from build123d import *

# Parameters (mm, degrees)
F0_W     = 140
F0_H     = 160
F1_DEPTH = 3.5
F2_W     = 31.75
F2_H     = 31.75
F2_W_2   = 25.4
F2_H_2   = 25.4
F3_DEPTH = 160
F4_W     = 25.4
F4_H     = 25.4
F4_W_2   = 19.4
F4_H_2   = 19.4
F5_DEPTH = 15
F6_R     = 3
F7_DEPTH = 4
F8_R     = 1
F9_DEPTH = 5


with BuildPart() as f1:
    # F0 (on Top) → F1 (new body)
    with BuildSketch(Plane.XY):
        with Locations((-1.276044, 37.026612)):
            Rectangle(F0_W, F0_H)
    extrude(amount=F1_DEPTH)

    # F2 (on face) → F3 (join)
    with BuildSketch(Plane.XZ.offset(42.973388)):
        with Locations((-55.401044, -15.875)):
            Rectangle(F2_W, F2_H)
        with Locations((-55.401044, -15.875)):
            Rectangle(F2_W_2, F2_H_2, mode=Mode.SUBTRACT)
        with Locations((52.848956, -15.875)):
            Rectangle(F2_W, F2_H)
        with Locations((52.848956, -15.875)):
            Rectangle(F2_W_2, F2_H_2, mode=Mode.SUBTRACT)
    extrude(amount=-F3_DEPTH)

    # F4 (on face) → F5 (join, symmetric)
    with BuildSketch(Plane.XZ.offset(42.973388)):
        with Locations((-55.401044, -15.875)):
            Rectangle(F4_W, F4_H)
        with Locations((-55.401044, -15.875)):
            Rectangle(F4_W_2, F4_H_2, mode=Mode.SUBTRACT)
        with Locations((52.848956, -15.875)):
            Rectangle(F4_W, F4_H)
        with Locations((52.848956, -15.875)):
            Rectangle(F4_W_2, F4_H_2, mode=Mode.SUBTRACT)
    extrude(amount=F5_DEPTH, both=True)

    # F6 (on face) → F7 (cut)
    with BuildSketch(Plane.YZ.offset(-39.526044)):
        with Locations((37.026612, -21.75)):
            Circle(F6_R)
    extrude(amount=-F7_DEPTH, mode=Mode.SUBTRACT)

    # F8 (on face) → F9 (cut)
    with BuildSketch(Plane.XY.offset(3.5)):
        with Locations((-66.276044, 112.026612)):
            Circle(F8_R)
        with Locations((63.723956, 112.026612)):
            Circle(F8_R)
        with Locations((63.723956, -37.973388)):
            Circle(F8_R)
        with Locations((-66.276044, -37.973388)):
            Circle(F8_R)
    extrude(amount=-F9_DEPTH, mode=Mode.SUBTRACT)


solid = f1.part
Design review of the part built by this model. Coordinates are the model's own, in mm. A direction names the side the tool comes from. Give positions to 0.01 mm unless a question says otherwise; leave off trailing zeros. Loops run counter-clockwise (first coordinate to the right, second up) from the corner with the lowest first, then second, coordinate; pieces in that order, holes last. Notation, with made-up numbers: (22, -24.75) - (70, -24.75) arc R21 cw to (70, -5.75) - close; hole circle Ø1 at (44.25, 51). An arc over 180 degrees is marked (long way). Write item = value, one per line.
1) Take a section at D-D on x = 0. State the section outline as (y, z) points, and give its area (3 significant figures).
Result sheet:
outline = (-42.97, 0) - (117.03, 0) - (117.03, 3.5) - (-42.97, 3.5) - close
area = 560 mm2
2) Clearance check with flat-ended pins moving along their axes: pin 1 Ø9.5 at (x, y) = (-54, -45.5) entering from +Z; pin 2 Ø7.5 at (x, y) = (46.5, -49) entering from -Z (3 decimals); pin 3 Ø2 at (x, z) = (35, -13) entering from +Y; pin 4 Ø0.6 at (x, y) = (63.5, 111.5) entering from +Z. State where each tip first meets the part, or that it passes through.
Result sheet:
pin_1 = 3.5
pin_2 = -28.575
pin_3 = through
pin_4 = -1.5
3) Take a section at A-A on z = -12.5. Count the separate pieces of the cut face and the enclosed holes in it, and give its area (3 significant figures).
Result sheet:
separate_pieces = 4
enclosed_holes = 0
area = 2,390 mm2
4) To check wall thickness, follow line 1 (X direction, y = 36, z = -19); line 2 (X direction, y = -50, z = -13); line 3 (X direction, y = 3.5, z = -10). State the ranges of each line that lie inside material, in increasing order.
Result sheet:
line_1 = -71.28 to -68.1, 36.97 to 40.15, 65.55 to 68.72
line_2 = -68.1 to -65.1, -45.7 to -42.7, 40.15 to 43.15, 62.55 to 65.55
line_3 = -71.28 to -68.1, -42.7 to -39.53, 36.97 to 40.15, 65.55 to 68.72
5) Draft analysis for pull direction Z (two halves, no side actions). For faces 1 (the face through (-56, -43, -6.175)), 2 (the face through (-65.101, -43, -16)), 3 (the face through (53, 36, -31.75)), 4 (the face through (68.724, 36, -14)), state which applies: +Z half, -Z half, draft (parallel to the pull), parting line (faces both ways), or undercut.
Result sheet:
face_1 = undercut
face_2 = undercut
face_3 = -Z half
face_4 = draft
6) Take a section at B-B on x = -57.5. State the section outline as (y, z) points (3 decimals).
Result sheet:
outline = (-57.973, -28.575) - (-42.973, -28.575) - (-42.973, -31.75) - (117.027, -31.75) - (117.027, -28.575) - (-27.973, -28.575) - (-27.973, -25.575) - (-57.973, -25.575) - close; (-57.973, -6.175) - (-27.973, -6.175) - (-27.973, -3.175) - (117.027, -3.175) - (117.027, 3.5) - (-42.973, 3.5) - (-42.973, -3.175) - (-57.973, -3.175) - close
7) Tool access review of faces 5 (the face through (62.549, -43, -16)), 6 (the face through (-41.091, 39.798, -22.899)), 7 (the face through (-56, 44, -28.575)), 8 (the face through (40.149, -51, -16)), 9 (the face through (36.974, 36, -16)): name each direction out of +Z, -Z, +X, -X, +Y, -Y from which nothing blocks a thin tool from reaching the whole face with its end or side.
Result sheet:
face_5 = +Y, -Y
face_6 = none
face_7 = +Y
face_8 = +Z, -Z, -Y
face_9 = -Z, +Y, -Y
8) Take a section at C-C on y = 80. State the section outline as (x, z) points (3 decimals).
Result sheet:
outline = (-71.276, -31.75) - (-39.526, -31.75) - (-39.526, 0) - (36.974, 0) - (36.974, -31.75) - (68.724, -31.75) - (68.724, 3.5) - (-71.276, 3.5) - close; hole (-68.101, -28.575) - (-42.701, -28.575) - (-42.701, -3.175) - (-68.101, -3.175) - close; hole (40.149, -28.575) - (65.549, -28.575) - (65.549, -3.175) - (40.149, -3.175) - close
